Work out the finished part from the listing and answer in its coordinate system (mm). Round coordinates to 2 decimals unless told otherwise and drop trailing zeros. Order: outer loops, then holes, each group sorted by start corner. A loop starts at its lowest first (then second) coordinate and runs counter-clockwise, first axis right, second up. Notation, with made-up numbers: (-12, 40) -> (32, 40) arc R33 ccw to (32, 69) -> close; hole circle Ø3 at (-35, 88.25). An arc over 180 degrees is marked (long way). Use a Markdown table: item, result. Add a question column.
Item 1: Find the intervals of material crossed by L1, parallel to Y at x = -88.5, z = 1.5; L2, parallel to Y at x = 9, z = 5.75; L3, parallel to X at y = 12, z = 3.75, in increasing order. Write a range as [from, to].
Item 2: For a pull along X with two mould halves and no side action, classify faces 1 (the cylindrical face through (-4.336, -19.524, 2.958)), 2 (the cylindrical face through (-93.65, 0.22, 2.96)), 3 (the flat face through (-35, 0, 0)), 4 (the cylindrical face through (32.492, 0.715, 2.958)) as +X half, -X half, draft (parallel to the pull), parting line (faces both ways), or undercut.
Item 3: A cutting plane is placed at D-D, the plane z = 4. Give the number of separate pieces and of enclosed holes in the cut face, plus the area to 3 significant figures.
Item 4: A cutting plane is placed at B-B, the plane x = 3.5. Determine the outline of the cut face in (y, z).
Item 5: A cutting plane is placed at A-A, the plane y = 0. Determine the outline of the cut face in (x, z).
Item 6: A cutting plane is placed at C-C, the plane y = -9. Determine the outline of the cut face in (x, z).
from build123d import *

# Parameters (mm, degrees)
SKETCH_1_R      = 20
SKETCH_1_R_2    = 5
EXTRUDE_1_DEPTH = 6


with BuildPart() as part:
    # Эскиз1 → Вытянуть1 (new body)
    with BuildSketch(Plane.XY):
        with BuildLine():
            Line((-88.652848771, 19.249029144), (0, 32.5))
            ThreePointArc((0, 32.5), (32.5, 0), (0, -32.5))
            add(Edge.make_bspline(
                [(-88.652848771, -17.726099374), (-70.912657014, -19.048471367), (-58.669056624, -9.575263386), (-25.513197615, -17.946964386), (-19.385232924, -31.623438469), (0, -32.5)],
                knots=[0, 0, 0, 0, 0.412174962, 0.512174962, 1, 1, 1, 1], degree=3))
            ThreePointArc((-88.652848771, -17.726099374), (-104.582448721, 0.761464885), (-88.652848771, 19.249029144))
        make_face()
        Circle(SKETCH_1_R, mode=Mode.SUBTRACT)
        with Locations((-88.652848771, 0)):
            Circle(SKETCH_1_R_2, mode=Mode.SUBTRACT)
    extrude(amount=EXTRUDE_1_DEPTH)


solid = part.part
Reported:
| question | item | result |
|---|---|---|
| 1 | L1 | [-17.74, -5], [5, 19.27] |
| 1 | L2 | [-31.23, -17.86], [17.86, 31.23] |
| 1 | L3 | [-100.83, -16], [16, 30.2] |
| 2 | face 1 | undercut |
| 2 | face 2 | undercut |
| 2 | face 3 | draft |
| 2 | face 4 | +X half |
| 3 | separate pieces | 1 |
| 3 | enclosed holes | 2 |
| 3 | area | 4,800 mm² |
| 4 | outline | (-32.31, 0) -> (-19.69, 0) -> (-19.69, 6) -> (-32.31, 6) -> close; (19.69, 0) -> (32.31, 0) -> (32.31, 6) -> (19.69, 6) -> close |
| 5 | outline | (-104.57, 0) -> (-93.65, 0) -> (-93.65, 6) -> (-104.57, 6) -> close; (-83.65, 0) -> (-20, 0) -> (-20, 6) -> (-83.65, 6) -> close; (20, 0) -> (32.5, 0) -> (32.5, 6) -> (20, 6) -> close |
| 6 | outline | (-101.83, 0) -> (-17.86, 0) -> (-17.86, 6) -> (-101.83, 6) -> close; (17.86, 0) -> (31.23, 0) -> (31.23, 6) -> (17.86, 6) -> close |
